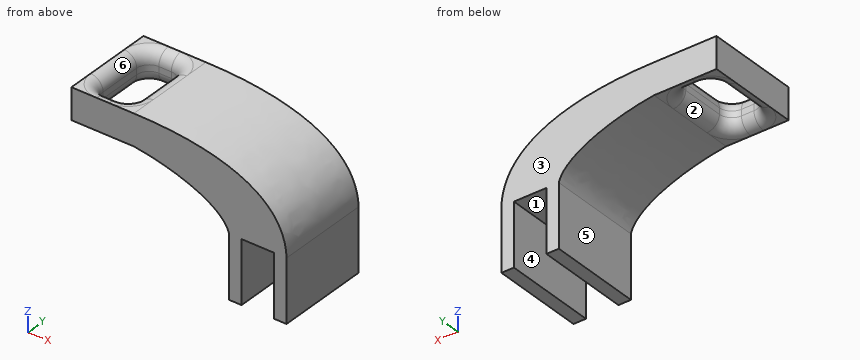
from build123d import *

# Parameters (mm, degrees)
F1_DEPTH = 19.05
F2_W     = 7.62
F2_H     = 13.97
F3_DEPTH = 6.35
F4_R     = 2.54
F5_R     = 2.53999
F6_R     = 2.53999


# Not quite as in the source:
# - a fillet or chamfer is up to 0.001 mm smaller than in the source, because OpenCascade refuses the exact size


with BuildPart() as f1:
    # F0 (on Front) → F1 (new body)
    with BuildSketch(Plane.XZ):
        with BuildLine():
            Line((-3.302, 6.35), (3.302, 6.35))
            Line((3.302, 6.35), (3.302, -6.35))
            Line((3.302, -6.35), (5.842, -6.35))
            Line((5.842, -6.35), (5.842, 6.35))
            add(Edge.make_bspline(
                [(-25.2045363516, 21.8299297452), (-6.6467649303, 21.8811389059), (5.5305822752, 17.0102007687), (5.842, 6.35)],
                knots=[0, 0, 0, 0, 34.6917229948, 34.6917229948, 34.6917229948, 34.6917229948], degree=3))
            Line((-25.2045363516, 21.8299297452), (-37.9045363516, 21.8299297452))
            Line((-37.9045363516, 21.8299297452), (-37.9045363516, 15.4799297452))
            Line((-37.9045363516, 15.4799297452), (-25.2045363516, 15.4799297452))
            add(Edge.make_bspline(
                [(-25.2045363516, 15.4799297452), (-17.7111625671, 14.5441424102), (-7.1151247248, 11.2962136045), (-5.842, 6.35)],
                knots=[0, 0, 0, 0, 21.4070883382, 21.4070883382, 21.4070883382, 21.4070883382], degree=3))
            Line((-5.842, 6.35), (-5.842, -6.35))
            Line((-5.842, -6.35), (-3.302, -6.35))
            Line((-3.302, -6.35), (-3.302, 6.35))
        make_face()
    extrude(amount=F1_DEPTH)

    # F2 (on face) → F3 (cut)
    with BuildSketch(Plane.XY.offset(21.8299297452)):
        with Locations((-31.5545363516, -9.525)):
            Rectangle(F2_W, F2_H)
    extrude(amount=-F3_DEPTH, mode=Mode.SUBTRACT)

    # F4
    f4_edges = [f1.edges().sort_by_distance(p)[0] for p in [
        (-27.744536, -2.54, 18.65493),
        (-35.364536, -2.54, 18.65493),
        (-35.364536, -16.51, 18.65493),
        (-27.744536, -16.51, 18.65493),
    ]]
    fillet(f4_edges, radius=F4_R)

    # F5 (radius 2.54 in the source; OpenCascade refuses exactly that, so slightly less here)
    f5_edges = [f1.edges().sort_by_distance(p)[0] for p in [
        (-35.364536, -9.525, 15.47993),
        (-34.620588, -15.766051, 15.47993),
        (-31.554536, -16.51, 15.47993),
        (-28.488485, -15.766051, 15.47993),
        (-27.744536, -9.525, 15.47993),
        (-31.554536, -2.54, 15.47993),
        (-34.620588, -3.283949, 15.47993),
        (-28.488485, -3.283949, 15.47993),
    ]]
    fillet(f5_edges, radius=F5_R)

    # F6 (radius 2.54 in the source; OpenCascade refuses exactly that, so slightly less here)
    f6_edges = [f1.edges().sort_by_distance(p)[0] for p in [
        (-31.554536, -16.51, 21.82993),
        (-34.620588, -15.766051, 21.82993),
        (-28.488485, -15.766051, 21.82993),
        (-35.364536, -9.525, 21.82993),
        (-27.744536, -9.525, 21.82993),
        (-28.488485, -3.283949, 21.82993),
        (-31.554536, -2.54, 21.82993),
        (-34.620588, -3.283949, 21.82993),
    ]]
    fillet(f6_edges, radius=F6_R)


solid = f1.part
Geometry: final body of the model. Coordinates: model frame, mm. Face numbers are marked on the shaded views. A direction names the side the tool comes from. Give positions to 0.01 mm unless a question says otherwise; leave off trailing zeros. Loops run counter-clockwise (first coordinate to the right, second up) from the corner with the lowest first, then second, coordinate; pieces in that order, holes last. Notation, with made-up numbers: (29, -21) -> (41, -21) arc R28 ccw to (41, 3) -> close; hole circle Ø2 at (65, 26.5). An arc over 180 degrees is marked (long way). Put each result on its own line as item: value.
1. Pin query (flat end, axial travel): P1, Ø10, axis at y = -8.5, z = 0, coming from the -X side; P2, Ø5.5, axis at x = -0.5, y = -7, coming from the -Z side; P3, Ø1, axis at y = -8.5, z = 18.5, coming from the +X side; P4, Ø3, axis at x = -7, y = -5, coming from the -Z side. Return the tip coordinate at first contact, or that it passes through.
Taken from the geometry:
P1: stops at x = -5.84
P2: stops at z = 6.35
P3: stops at x = -2.62
P4: stops at z = -6.35
2. Cut plane A-A (z = 5.5). Return the cut outline in (x, y).
Taken from the geometry:
outline: (-5.84, -19.05) -> (-3.3, -19.05) -> (-3.3, 0) -> (-5.84, 0) -> close; (3.3, -19.05) -> (5.84, -19.05) -> (5.84, 0) -> (3.3, 0) -> close
3. Ray query, line 1 along X through (y, z) = (-3, -0.75); line 2 along X through (y, z) = (-9, 17.75); line 3 along Z through (x, y) = (-24.5, -9.5). Return the intervals inside material, ascending. Write a range as [from, to].
Taken from the geometry:
line 1: x = [-5.84, -3.3], [3.3, 5.84]
line 2: x = [-37.9, -35.38], [-27.73, -2.11]
line 3: z = [15.39, 21.83]
4. Pull-direction query (Y, two-part tool) for the marked faces 1, 2 and 3; classes: released by +Y, released by -Y, zero draft, split by the parting line, or undercut.
Taken from the geometry:
face 1: zero draft
face 2: undercut
face 3: released by +Y
5. Set-up query: the marked faces 4, 5 and 6. Return all of +Z, -Z, +X, -X, +Y, -Y with unobstructed straight access to the full face (end or side cutting, diameter ignored); none if empty.
Taken from the geometry:
face 4: -Z, +Y, -Y
face 5: -Z, -X, +Y, -Y
face 6: +Z
